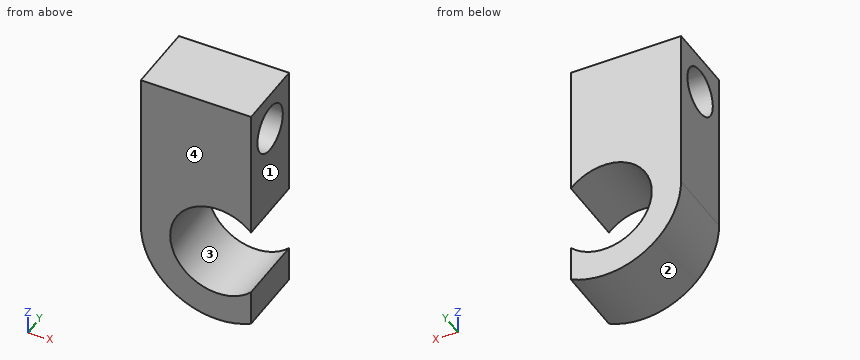
```python
from build123d import *

# Parameters (mm, degrees)
BOSS_EXTRUDE1_DEPTH = 9.525
BOSS_EXTRUDE2_DEPTH = 9.525
SKETCH3_R           = 3.175
CUT_EXTRUDE1_DEPTH  = 15.774697863


with BuildPart() as part:
    # Sketch1 → Boss-Extrude1 (new body)
    with BuildSketch(Plane(origin=(0, 0, 0), x_dir=(1, 0, 0), z_dir=(0, 1, 0))):
        with BuildLine():
            Line((4.490128061, 4.490128061), (4.490128061, 9.252628061))
            ThreePointArc((4.490128061, 9.252628061), (-10.284569803, 0), (4.490128061, -9.252628061))
            Line((4.490128061, -9.252628061), (4.490128061, -4.490128061))
            ThreePointArc((4.490128061, -4.490128061), (-6.35, 0), (4.490128061, 4.490128061))
        make_face()
    extrude(amount=BOSS_EXTRUDE1_DEPTH)

    # Sketch2 → Boss-Extrude2 (add, through all)
    with BuildSketch(Plane(origin=(0, 9.525, 0), x_dir=(1, 0, 0), z_dir=(0, 1, 0))):
        with BuildLine():
            Line((-10.284569803, 0), (-10.284569803, -21.952628061))
            Line((-10.284569803, -21.952628061), (4.490128061, -21.952628061))
            Line((4.490128061, -21.952628061), (4.490128061, -9.252628061))
            ThreePointArc((4.490128061, -9.252628061), (-5.458632639, -8.716404405), (-10.284569803, 0))
        make_face()
    extrude(amount=-BOSS_EXTRUDE2_DEPTH)

    # Sketch3 → Cut-Extrude1 (cut, through all)
    with BuildSketch(Plane.ZY.offset(10.284569803)):
        with Locations((16.872628061, 4.7625)):
            Circle(SKETCH3_R)
    extrude(amount=-CUT_EXTRUDE1_DEPTH, mode=Mode.SUBTRACT)


solid = part.part
```
Geometry: final body of the model. Coordinates: model frame, mm. Face numbers are marked on the shaded views. Coordinates: 2 decimals unless noted, no trailing zeros. Order: outer loops, then holes, each group sorted by start corner. A loop starts at its lowest first (then second) coordinate and runs counter-clockwise, first axis right, second up. Notation, with made-up numbers: M -36.75,54.5 L -30.75,54.5 A24 cw -30.75,73.5 Z; hole C 27.25,87.5 d1. An arc over 180 degrees is marked long. Answer as CSV lines item,"result".
Q1. Section A-A on x = 0. Count the separate pieces of the cut face and the enclosed holes in it, and give its area (3 significant figures).
Answers:
separate pieces,"2"
enclosed holes,"1"
area,"154 mm^2"
Q2. Section C-C on z = 5.5. Return the cut outline in (x, y) (3 decimals).
Answers:
outline,"M -10.285,0 L -3.174,0 L -3.174,9.525 L -10.285,9.525 Z; M 3.174,0 L 4.49,0 L 4.49,9.525 L 3.174,9.525 Z"
Q3. Line query: probe 1 along Z at (x, y) = (0, 5.75); probe 2 along Z at (x, y) = (0, 4.25); probe 3 along Y at (x, z) = (-2.75, 18) (3 decimals). Output: solid intervals per line, ascending. Write a range as [from, to].
Answers:
probe 1,"z = [-10.28, -6.35], [6.35, 13.86], [19.89, 21.95]"
probe 2,"z = [-10.28, -6.35], [6.35, 13.74], [20.01, 21.95]"
probe 3,"y = [0, 1.794], [7.731, 9.525]"
Q4. Section B-B on y = 5.75. Return the cut outline in (x, z).
Answers:
outline,"M -10.28,0 A10.28 ccw 4.49,-9.25 L 4.49,-4.49 A6.35 cw long 4.49,4.49 L 4.49,13.86 L -10.28,13.86 Z; M -10.28,19.89 L 4.49,19.89 L 4.49,21.95 L -10.28,21.95 Z"
Q5. Draft query along X for the marked faces 1, 2, 3 and 4. Return one class per face: pulls with the +X half, pulls with the -X half, needs draft (parallel to the pull), parting line crosses it, or undercut.
Answers:
face 1,"pulls with the +X half"
face 2,"parting line crosses it"
face 3,"undercut"
face 4,"needs draft"
Q6. First-contact query: P1, Ø5, axis at y = 4.76, z = 16.87, coming from the +X side; P2, Ø3, axis at y = 7, z = 1.5, coming from the +X side. Flat tips, straight axial feed; report the tip coordinate or a pass-through.
Answers:
P1,"passes through"
P2,"stops at x = -5.6"
